```python
from build123d import *

# Parameters (mm, degrees)
SCHIZZO2_W                = 95.661065857
SCHIZZO2_H                = 99.914617901
SCHIZZO2_W_2              = 85.661065857
SCHIZZO2_H_2              = 89.914617901
ESTRUSIONE_SOTTILE1_DEPTH = 45
SCHIZZO5_W                = 14.572404991
SCHIZZO5_H                = 31.877712984
TAGLIO_ESTRUSIONE2_DEPTH  = 5
SCHIZZO6_W                = 17.563316518
SCHIZZO6_H                = 14.837974299
SCHIZZO6_W_2              = 14.53926904
SCHIZZO6_H_2              = 16.284185158
SCHIZZO6_W_3              = 14.178791295
TAGLIO_ESTRUSIONE3_DEPTH  = 5
SMUSSO5_SIZE              = 2
SMUSSO6_SIZE              = 1.5
SKETCH1_R                 = 6
SKETCH1_W                 = 24.285177085
SKETCH1_H                 = 14.972609064
CUT_EXTRUDE1_DEPTH        = 10
FILLET1_R                 = 2
FILLET2_R                 = 1
SKETCH2_W                 = 95.661065857
SKETCH2_H                 = 99.914617901
BOSS_EXTRUDE1_DEPTH       = 4


with BuildPart() as part:
    # Schizzo2 → Estrusione-Sottile1 (new body)
    with BuildSketch(Plane.XY.offset(6.703232706)):
        with Locations((-1.032219499, 3.65730895)):
            Rectangle(SCHIZZO2_W, SCHIZZO2_H)
        with Locations((-1.032219499, 3.65730895)):
            Rectangle(SCHIZZO2_W_2, SCHIZZO2_H_2, mode=Mode.SUBTRACT)
    extrude(amount=-ESTRUSIONE_SOTTILE1_DEPTH)

    # Schizzo5 → Taglio-Estrusione2 (cut)
    with BuildSketch(Plane(origin=(46.798313429, 0, 0), x_dir=(0, 0, -1), z_dir=(1, 0, 0))):
        Polygon((32.751075083, 35.734689364), (24.713552886, 35.734689364), (24.713552886, 19.705476421), (17.402976387, 19.705476421), (17.402976387, 5.715425641), (11.875438841, 5.715425641), (11.875438841, 5.226263026), (11.875438841, -4.850486837), (24.713552886, -4.850486837), (24.713552886, 5.470844333), (29.271954363, 5.470844333), (29.271954363, 15.813468704), (32.751075083, 15.813468704), align=None)
        with Locations((19.448395228, -25.361143508)):
            Rectangle(SCHIZZO5_W, SCHIZZO5_H)
    extrude(amount=-TAGLIO_ESTRUSIONE2_DEPTH, mode=Mode.SUBTRACT)

    # Schizzo6 → Taglio-Estrusione3 (cut)
    with BuildSketch(Plane.XZ.offset(46.3)):
        with Locations((18.323185023, -16.793891295)):
            Rectangle(SCHIZZO6_W, SCHIZZO6_H)
        with Locations((-6.016266439, -16.070785866)):
            Rectangle(SCHIZZO6_W_2, SCHIZZO6_H_2)
        with Locations((-28.245727369, -16.070785866)):
            Rectangle(SCHIZZO6_W_3, SCHIZZO6_H_2)
    extrude(amount=-TAGLIO_ESTRUSIONE3_DEPTH, mode=Mode.SUBTRACT)

    # Smusso5
    smusso5_edges = [part.edges().sort_by_distance(p)[0] for p in [
        (-35.335123016, -46.3, -16.070785866),
        (-28.245727368, -46.3, -24.212878445),
        (-21.156331721, -46.3, -16.070785866),
        (-28.245727368, -46.3, -7.928693287),
    ]]
    chamfer(smusso5_edges, length=SMUSSO5_SIZE)

    # Smusso6
    smusso6_edges = [part.edges().sort_by_distance(p)[0] for p in [
        (46.798313429, 25.774079034, -32.751075083),
    ]]
    chamfer(smusso6_edges, length=SMUSSO6_SIZE)

    # Sketch1 → Cut-Extrude1 (cut)
    with BuildSketch(Plane(origin=(0, 53.614617901, 0), x_dir=(1, 0, 0), z_dir=(0, 1, 0))):
        with Locations(Location((20.937247572, 21.021954363, 0), (0, 0, 270))):
            Circle(SKETCH1_R)
        with Locations(Location((6.937247572, 21.021954363, 0), (0, 0, 270))):
            Circle(SKETCH1_R)
        with Locations((-27.662752428, 21.785649831)):
            Rectangle(SKETCH1_W, SKETCH1_H)
    extrude(amount=-CUT_EXTRUDE1_DEPTH, mode=Mode.SUBTRACT)

    # Fillet1
    fillet1_edges = [part.edges().sort_by_distance(p)[0] for p in [
        (1.253368081, -46.3, -16.070785866),
        (-6.016266439, -46.3, -7.928693287),
        (-13.285900959, -46.3, -16.070785866),
        (-6.016266439, -46.3, -24.212878445),
    ]]
    fillet(fillet1_edges, radius=FILLET1_R)

    # Fillet2
    fillet2_edges = [part.edges().sort_by_distance(p)[0] for p in [
        (9.541526764, -46.3, -16.793891295),
        (18.323185023, -46.3, -24.212878445),
        (27.104843282, -46.3, -16.793891295),
        (18.323185023, -46.3, -9.374904146),
    ]]
    fillet(fillet2_edges, radius=FILLET2_R)

    # Sketch2 → Boss-Extrude1 (add)
    with BuildSketch(Plane.XY.offset(6.703232706)):
        with Locations((-1.032219499, 3.65730895)):
            Rectangle(SKETCH2_W, SKETCH2_H)
    extrude(amount=BOSS_EXTRUDE1_DEPTH)


solid = part.part
```
Design review of the part built by this model. Coordinates are the model's own, in mm. A direction names the side the tool comes from. Round coordinates to 2 decimals unless told otherwise and drop trailing zeros. Write each loop counter-clockwise with the first axis right and the second up, starting at its lowest first coordinate (ties: lowest second). Pieces come first, ordered by that corner, then holes. Notation, with made-up numbers: (20.25, 10) -> (79.25, 10) arc R20 ccw to (79.25, 48) -> close; hole circle Ø6 at (-35, 20.5). An arc over 180 degrees is marked (long way). Answer in a Markdown table with one row per item.
Q1. For faces 3 (the face through (-21.156, -43, -16)), 4 (the face through (44, 35.735, -30)), 5 (the face through (-39.805, 51, -22)), 6 (the face through (-28, -43, -24.213)), 7 (the face through (41.798, 3, -10)), list the 3-axis set-ups (+Z, -Z, +X, -X, +Y, -Y) from which the entire face can be reached by the end or side of a thin tool; tool diameter is ignored.
The answers:
| item | result |
|---|---|
| face 3 | -Y |
| face 4 | +X |
| face 5 | +Y |
| face 6 | +Y, -Y |
| face 7 | -Z |
Q2. Take a section at A-A, the plane x = -33.5. State the section outline as (y, z) points, then the cut area to 3 significant figures.
The answers:
| item | result |
|---|---|
| outline | (-46.3, -38.3) -> (-41.3, -38.3) -> (-41.3, -24.21) -> (-44.3, -24.21) -> (-46.3, -26.21) -> close; (-46.3, -5.93) -> (-44.3, -7.93) -> (-41.3, -7.93) -> (-41.3, 6.7) -> (48.61, 6.7) -> (48.61, -14.3) -> (53.61, -14.3) -> (53.61, 10.7) -> (-46.3, 10.7) -> close; (48.61, -38.3) -> (53.61, -38.3) -> (53.61, -29.27) -> (48.61, -29.27) -> close |
| area | 689 mm² |
Q3. To check wall thickness, follow L1, parallel to X at y = 34, z = -20.5; L2, parallel to Y at x = -18, z = 3; L3, parallel to Z at x = 11, y = 21.5. State the ranges of each line that lie inside material, in increasing order. Write a range as [from, to].
The answers:
| item | result |
|---|---|
| L1 | [-48.86, -43.86], [41.8, 46.8] |
| L2 | [-46.3, -41.3], [48.61, 53.61] |
| L3 | [6.7, 10.7] |
Q4. Take a section at C-C, the plane z = 4. State the section outline as (x, y) points.
The answers:
| item | result |
|---|---|
| outline | (-48.86, -46.3) -> (46.8, -46.3) -> (46.8, 53.61) -> (-48.86, 53.61) -> close; hole (-43.86, -41.3) -> (41.8, -41.3) -> (41.8, 48.61) -> (-43.86, 48.61) -> close |
Q5. Take a section at D-D, the plane x = -10.5. State the section outline as (y, z) points, then the cut area to 3 significant figures.
The answers:
| item | result |
|---|---|
| outline | (-46.3, -38.3) -> (-41.3, -38.3) -> (-41.3, -24.21) -> (-44.3, -24.21) arc R2 ccw to (-46.3, -26.21) -> close; (-46.3, -5.93) arc R2 ccw to (-44.3, -7.93) -> (-41.3, -7.93) -> (-41.3, 6.7) -> (48.61, 6.7) -> (48.61, -38.3) -> (53.61, -38.3) -> (53.61, 10.7) -> (-46.3, 10.7) -> close |
| area | 767 mm² |
Q6. Take a section at B-B, the plane y = 26. State the section outline as (x, z) points.
The answers:
| item | result |
|---|---|
| outline | (-48.86, -38.3) -> (-43.86, -38.3) -> (-43.86, 6.7) -> (41.8, 6.7) -> (41.8, -24.71) -> (46.8, -24.71) -> (46.8, 10.7) -> (-48.86, 10.7) -> close; (41.8, -38.3) -> (46.8, -38.3) -> (46.8, -34.25) -> (45.3, -32.75) -> (41.8, -32.75) -> close |
Q7. Clearance check with flat-ended pins moving along their axes: pin 1 Ø3 at (x, y) = (1.5, -19.5) entering from -Z; pin 2 Ø9.5 at (x, z) = (20.94, -21.02) entering from +Y; pin 3 Ø1.5 at (x, z) = (16.5, -24) entering from -Y. State where each tip first meets the part, or that it passes through.
The answers:
| item | result |
|---|---|
| pin 1 | z = 6.7 |
| pin 2 | y = -41.3 |
| pin 3 | y = -46.19 |
Q8. Draft analysis for pull direction Z (two halves, no side actions). For faces 1 (the face through (-48.863, 3, -14)), 2 (the face through (1.253, -43, -16)), state which applies: +Z half, -Z half, draft (parallel to the pull), parting line (faces both ways), or undercut.
The answers:
| item | result |
|---|---|
| face 1 | draft |
| face 2 | undercut |
